Verification items for this drawing (mm, ordinates from the low corner). Round coordinates to 2 decimals unless told otherwise and drop trailing zeros. Order: outer loops, then holes, each group sorted by start corner. A loop starts at its lowest first (then second) coordinate and runs counter-clockwise, first axis right, second up. Notation, with made-up numbers: (18.5, 8.25) -> (44.5, 8.25) arc R34 cw to (44.5, 39.25) -> close; hole circle Ø2 at (35, 43). An arc over 180 degrees is marked (long way). Answer in a Markdown table with one row per item. Add a question column.
1. Sectioned sample at D-D, the plane z = 2. Record the boundary of the cut face in (x, y), then the cut area to 3 significant figures.
2. Sectioned sample at A-A, the plane z = 11.5. Record the boundary of the cut face in (x, y), then the cut area to 3 significant figures.
3. Sectioned sample at C-C, the plane x = 18. Record the boundary of the cut face in (y, z).
4. Draft check along X on the marked faces 1, 2, 3 and 4. Enter one of: +X half, -X half, draft (parallel to the pull), parting line (faces both ways), or undercut.
5. Material ranges on L1, parallel to X at y = 18.5, z = 12.5; L2, parallel to Y at x = 14.5, z = 4.75; L3, parallel to Y at x = 23.5, z = 4.75, recorded low to high. Write a range as from..to.
6. Depth check by flat-ended pin: P1, Ø2, axis at y = 33.5, z = 3, coming from the -X side; P2, Ø2, axis at y = 39, z = 13.5, coming from the +X side; P3, Ø0.6, axis at y = 38.5, z = 12, coming from the -X side. Enter the tip coordinate at first touch or a pass-through.
7. Sectioned sample at B-B, the plane y = 5. Record the boundary of the cut face in (x, z), then the cut area to 3 significant figures.
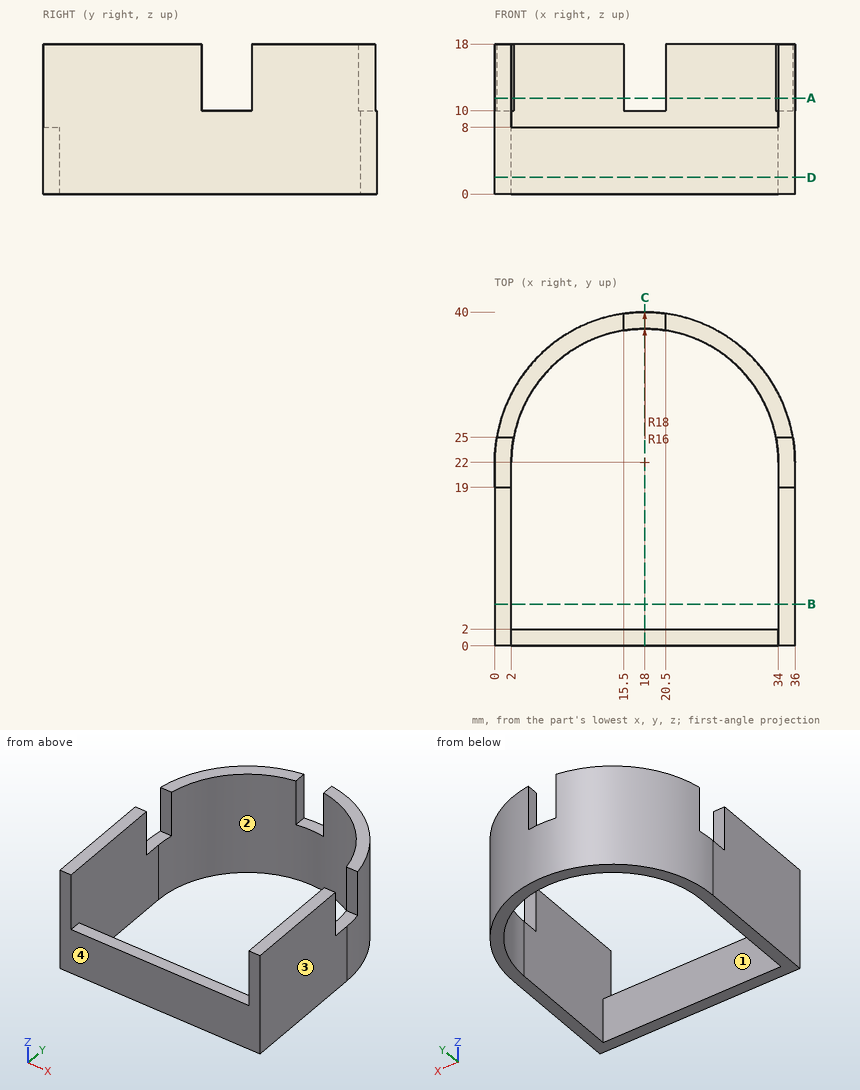
Answer key:
| question | item | result |
|---|---|---|
| 1 | outline | (0, 0) -> (36, 0) -> (36, 22) arc R18 ccw to (0, 22) -> close; hole (2, 2) -> (34, 2) -> (34, 22) arc R16 ccw to (2, 22) -> close |
| 1 | area | 259 mm² |
| 2 | outline | (0, 0) -> (2, 0) -> (2, 19) -> (0, 19) -> close; (0.25, 25) -> (2.28, 25) arc R16 cw to (15.5, 37.8) -> (15.5, 39.83) arc R18 ccw to start; (20.5, 37.8) arc R16 cw to (33.72, 25) -> (35.75, 25) arc R18 ccw to (20.5, 39.83) -> close; (34, 0) -> (36, 0) -> (36, 19) -> (34, 19) -> close |
| 2 | area | 161 mm² |
| 3 | outline | (0, 0) -> (2, 0) -> (2, 8) -> (0, 8) -> close; (38, 0) -> (40, 0) -> (40, 10) -> (38, 10) -> close |
| 4 | face 1 | undercut |
| 4 | face 2 | undercut |
| 4 | face 3 | +X half |
| 4 | face 4 | draft |
| 5 | L1 | x = 0..2, 34..36 |
| 5 | L2 | y = 0..2, 37.61..39.66 |
| 5 | L3 | y = 0..2, 37.02..39.14 |
| 6 | P1 | stops at x = 3.38 |
| 6 | P2 | stops at x = 26.25 |
| 6 | P3 | stops at x = 10.15 |
| 7 | outline | (0, 0) -> (2, 0) -> (2, 18) -> (0, 18) -> close; (34, 0) -> (36, 0) -> (36, 18) -> (34, 18) -> close |
| 7 | area | 72.0 mm² |
